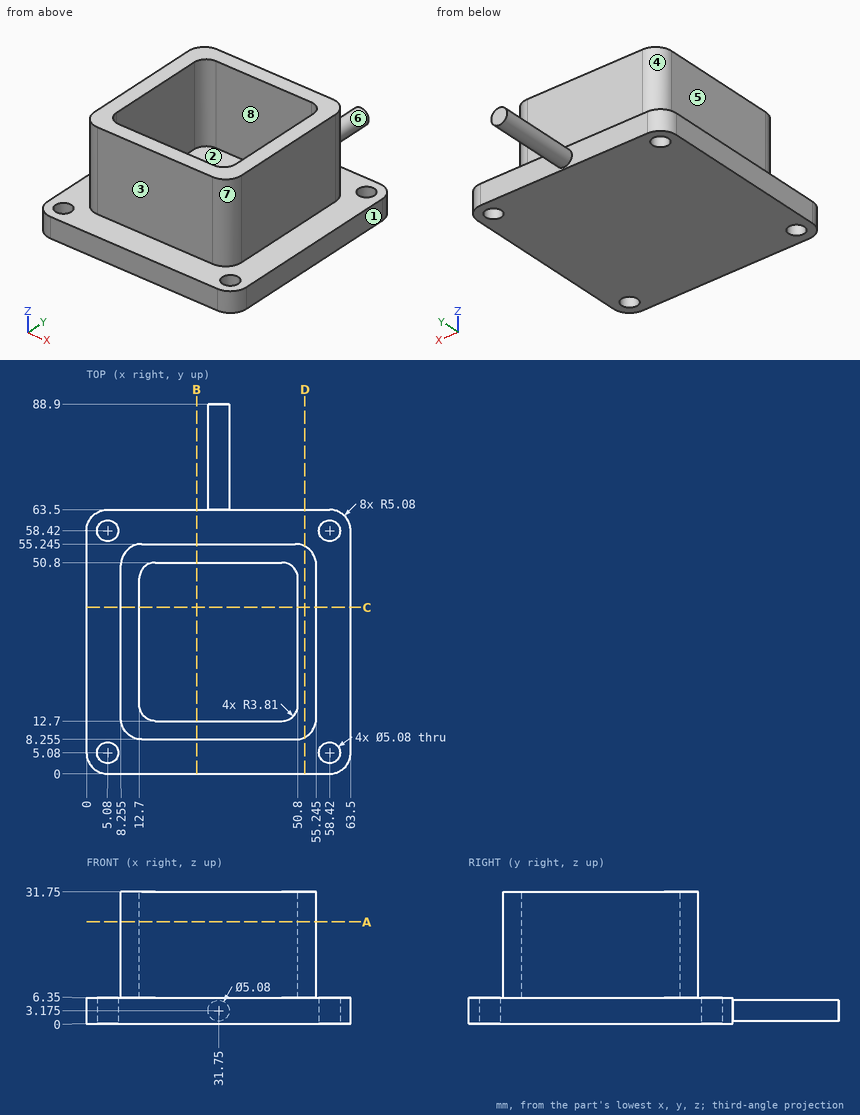
Study the drawing (mm; zero at the part's minimum x, y, z) and answer. A direction names the side the tool comes from. Give positions to 0.01 mm unless a question says otherwise; leave off trailing zeros. Order: outer loops, then holes, each group sorted by start corner. A loop starts at its lowest first (then second) coordinate and runs counter-clockwise, first axis right, second up. Notation, with made-up numbers: (80.5, 60) -> (125.5, 60) arc R22 ccw to (125.5, 84) -> close; hole circle Ø7 at (-18, 6.5). An arc over 180 degrees is marked (long way). Put each result on its own line as item: value.
Item 1: A cutting plane is placed at D-D on x = 52.5. Give the vertices of the cut face in (y, z), plus the area to 3 significant figures.
Established:
outline: (0, 0) -> (63.5, 0) -> (63.5, 6.35) -> (54.68, 6.35) -> (54.68, 31.75) -> (8.82, 31.75) -> (8.82, 6.35) -> (0, 6.35) -> close
area: 1,570 mm^2
Item 2: For the marked faces 4, 5, 6, 7 and 8, determine the directions among +Z, -Z, +X, -X, +Y, -Y from which every point of the face is accessible in a straight line to the end or side of a thin tool.
Established:
face 4: +Z, -X, +Y
face 5: +Z, -X, +Y, -Y
face 6: +Y
face 7: +Z, +X, -Y
face 8: +Z
Item 3: A cutting plane is placed at A-A on z = 24.5. Give the vertices of the cut face in (x, y) (3 decimals), plus the area to 3 significant figures.
Established:
outline: (8.255, 13.335) arc R5.08 ccw to (13.335, 8.255) -> (50.165, 8.255) arc R5.08 ccw to (55.245, 13.335) -> (55.245, 50.165) arc R5.08 ccw to (50.165, 55.245) -> (13.335, 55.245) arc R5.08 ccw to (8.255, 50.165) -> close; hole (12.7, 16.51) arc R3.81 ccw to (16.51, 12.7) -> (46.99, 12.7) arc R3.81 ccw to (50.8, 16.51) -> (50.8, 46.99) arc R3.81 ccw to (46.99, 50.8) -> (16.51, 50.8) arc R3.81 ccw to (12.7, 46.99) -> close
area: 747 mm^2
Item 4: Straight lines are drawn through the part: line 1 (Y direction, x = 37.5, z = 26) (3 decimals); line 2 (Y direction, x = 58.42, z = 2.5); line 3 (X direction, y = 58, z = 2). For each, find the intervals that lie inside material, in ascending order.
Established:
line 1: y = 8.255 to 12.7, 50.8 to 55.245
line 2: y = 0 to 2.54, 7.62 to 55.88, 60.96 to 63.5
line 3: x = 0 to 2.57, 7.59 to 55.91, 60.93 to 63.5
Item 5: Given P1, Ø4, axis at y = 17, z = 25.5, coming from the +X side (3 decimals); P2, Ø5, axis at x = 19.5, z = 2.5, coming from the +Y side; P3, Ø12, axis at x = 38.5, y = 35.5, coming from the +Z side; P4, Ø4.5, axis at x = 5.08, y = 5.08, coming from the -Z side, each flat-ended and moving along its own axis, determine where each tip first touches the part or whether it passes through.
Established:
P1: stops at x = 55.245
P2: stops at y = 63.5
P3: stops at z = 6.35
P4: passes through
Item 6: A cutting plane is placed at B-B on x = 26.5. Give the vertices of the cut face in (y, z) (3 decimals).
Established:
outline: (0, 0) -> (63.5, 0) -> (63.5, 6.35) -> (55.245, 6.35) -> (55.245, 31.75) -> (50.8, 31.75) -> (50.8, 6.35) -> (12.7, 6.35) -> (12.7, 31.75) -> (8.255, 31.75) -> (8.255, 6.35) -> (0, 6.35) -> close
Item 7: For a pull along Y with two mould halves and no side action, classify the marked faces 1, 2 and 3 as released by +Y, released by -Y, zero draft, split by the parting line, or undercut.
Established:
face 1: zero draft
face 2: undercut
face 3: released by -Y
